Geometry: final body of the model. Coordinates: model frame, mm. A direction names the side the tool comes from. Give positions to 0.01 mm unless a question says otherwise; leave off trailing zeros. Write each loop counter-clockwise with the first axis right and the second up, starting at its lowest first coordinate (ties: lowest second). Pieces come first, ordered by that corner, then holes.
Q1. Line query: line 1 (Y direction, x = 11, z = -35); line 2 (Y direction, x = 27.5, z = 35); line 3 (Z direction, x = 8.5, y = 14.5). Output: solid intervals per line, ascending.
Q2. Section C-C (y = 21.5). State how many separate pieces and enclosed holes the cut face has, plus the area to 3 significant figures.
Q3. Mould query, pull axis Y, two halves, no side actions, for faces 1 (the flat face through (9, 27, 1)), 2 (the cylindrical face through (26.1, 5.2, 39.4)), 3 (the flat face through (22, 17, 35)), 4 (the flat face through (0, 13, 35)). Classes: +Y half, -Y half, draft (parallel to the pull), parting line (faces both ways), or undercut.
Q4. Section A-A (x = 25.5). Return the cut outline in (y, z), plus the area to 3 significant figures.
Q5. Pin query (flat end, axial travel): pin 1 Ø3 at (y, z) = (19, -5) entering from -X; pin 2 Ø10 at (y, z) = (20.5, -35) entering from +X; pin 3 Ø7.5 at (y, z) = (16.5, 3) entering from +X. Return the tip coordinate at first contact, or that it passes through.
Q6. Section D-D (z = 5). Return the cut outline in (x, y), plus the area to 3 significant figures.
Q7. Reachability of faces 5 (the flat face through (15, 20, 10.5)), 6 (the flat face through (4, 13, 25.25)), 7 (the flat face through (22, 21, -39)) from +Z, -Z, +X, -X, +Y, -Y: full face, straight path, thin tool, end or side. Return the list, or none.
Q8. Section B-B (z = 35). Return the cut outline in (x, y), plus the area to 3 significant figures.
Autodesk Inventor part; units mm, degrees
ref_plane "YZ Plane" through (0, 0, 0) normal (1, 0, 0) x (0, 1, 0)
ref_plane "XZ Plane" through (0, 0, 0) normal (0, 1, 0) x (-1, 0, 0)
ref_plane "XY Plane" through (0, 0, 0) normal (0, 0, 1) x (1, 0, 0)
sketch "Szkic2" plane through (0, 0, 0) normal (0, 1, 0) x (-1, 0, 0)
  line L0 (-5, 13) -> (-5, -13)
  line L1 (1, -20.25) -> (1, 20.25)
  line L2 (-8.0627, 14.7682) -> (-5, 13)
  line L3 (-5, 16.0869) -> (-5, 13) construction
  arc A0 (-8.0627, 14.7682) -> (-5, 16.0869) centre (-8.5, 20) ccw construction
  line L4 (-3.256, 20.25) -> (-5, 20.25) construction
  arc A1 (-5, 16.0869) -> (-3.256, 20.25) centre (-8.5, 20) ccw construction
  line L5 (1, 20.25) -> (-3.256, 20.25)
  line L6 (-5, 20.25) -> (-5, 16.0869) construction
  line L7 (-5, -13) -> (-8.0627, -14.7682)
  line L8 (-5, -13) -> (-5, -16.0869) construction
  arc A2 (-5, -16.0869) -> (-8.0627, -14.7682) centre (-8.5, -20) ccw construction
  line L9 (-3.256, -20.25) -> (1, -20.25)
  arc A3 (-3.256, -20.25) -> (-5, -16.0869) centre (-8.5, -20) ccw construction
  line L10 (-5, -16.0869) -> (-5, -20.25) construction
  line L11 (-5, -20.25) -> (-3.256, -20.25) construction
  arc A4 (-8.0627, -14.7682) -> (-3.256, -20.25) centre (-8.5, -20) ccw
  arc A5 (-3.256, 20.25) -> (-8.0627, 14.7682) centre (-8.5, 20) ccw
  line L12 (0, 45) -> (-30, 45)
  line L13 (-30, 45) -> (-30, -45)
  line L14 (-30, -45) -> (0, -45)
  line L15 (0, -45) -> (0, 45)
  line L16 (-8.5, 25.25) -> (0, 25.25)
  line L17 (-8.5, -25.25) -> (0, -25.25)
  point P0 (0, 0)
  point P1 (0, -20.25)
  point P2 (0, 20.25)
  dimension "d0" = 10.5
  dimension "d1" = 6
  dimension "d2" = 3.5
  dimension "d3" = 120
  dimension "d4" = 120
  dimension "d5" = 26
  dimension "d6" = 40
  dimension "d8" = 7
  dimension "d9" = 0.25
  dimension "d10" = 0.25
  dimension "d12" = 9.5
  dimension "d14" = 1
  dimension "d15" = 20
  dimension "d16" = 90
  dimension "d17" = 45
  dimension "d18" = 30
extrude "Wyciągnięcie proste1" add sketch "Szkic2" along normal blind 27 contours L0 L7 A4 L17 L15 L14 L13 L12 L16 A5 L2
sketch "Szkic3" plane through (30, 0, 45) normal (1, 0, 0) x (0, 0, -1)
  circle A0 centre (10, 20.5) radius 3.25
  circle A1 centre (10, 8.5) radius 3.25
  circle A2 centre (80, 20.5) radius 3.25
  circle A3 centre (80, 8.5) radius 3.25
  line L0 (0, 0) -> (0, 27)
  line L1 (0, 27) -> (90, 27)
  line L2 (90, 0) -> (90, 27)
  circle A4 centre (10, 20.5) radius 5.5
  circle A5 centre (10, 8.5) radius 5.5
  circle A6 centre (80, 20.5) radius 5.5
  circle A7 centre (80, 8.5) radius 5.5
  point P0 (45, 0)
  dimension "d21" = 6.5
  dimension "d22" = 10
  dimension "d23" = 6.5
  dimension "d24" = 12
  dimension "d25" = 10
  dimension "d26" = 11
extrude "Wyciągnięcie proste2" cut sketch "Szkic3" against normal through all contours A0 | A1 | A2 | A3
extrude "Wyciągnięcie proste3" cut sketch "Szkic3" against normal blind 8 contours A1 | A2 | A3 | A4 | A5 | A6 | A7
sketch "Szkic4" plane through (0, 27, 0) normal (0, 1, 0) x (1, 0, 0)
  line L0 (30, -45) -> (30, 45)
  circle A0 centre (38.5, 0) radius 22
  point P0 (0, 0)
  dimension "d34" = 44
  dimension "d37" = 8.5
  dimension "d38" = 38.5
extrude "Wyciągnięcie proste4" cut sketch "Szkic4" against normal through all
sketch "Szkic8" plane through (0, 27, 0) normal (0, 1, 0) x (1, 0, 0)
  line L0 (11, -10.5) -> (21, -10.5)
  line L1 (21, -10.5) -> (21, 10.5)
  line L2 (21, 10.5) -> (11, 10.5)
  line L3 (11, 10.5) -> (11, -10.5)
  line L4 (5, 13) -> (5, -13)
  point P0 (0, 0)
  dimension "d58" = 21
  dimension "d59" = 6
  dimension "d60" = 10.5
  dimension "d61" = 10
extrude "Wyciągnięcie proste8" cut sketch "Szkic8" against normal blind 15
sketch "Szkic9" plane through (11, 27, 10.5) normal (1, 0, 0) x (0, 0, -1)
  circle A0 centre (5.5, -8) radius 1
  circle A1 centre (15.5, -8) radius 1
  line L0 (0, 0) -> (21, 0)
  line L1 (0, -15) -> (0, 0)
  point P0 (10.5, -27)
  dimension "d64" = 2
  dimension "d65" = 10
  dimension "d66" = 8
  dimension "d67" = 5.5
extrude "Wyciągnięcie proste9" cut sketch "Szkic9" against normal through all
equation "\"d25\" = d22"
properties part number "YCarriageFrontHolder" material "Tworzywo sztuczne ABS"
Computed:
1. line 1: y = 0 to 5.25, 11.75 to 17.25, 23.75 to 27
1. line 2: y = 0 to 3, 14 to 15, 26 to 27
1. line 3: z = -45 to -25.25, -14.75 to 14.75, 25.25 to 45
2. separate pieces: 3
2. enclosed holes: 0
2. area: 1,310 mm2
3. face 1: +Y half
3. face 2: undercut
3. face 3: undercut
3. face 4: draft
4. outline: (0, -45) - (27, -45) - (27, -17.75) - (0, -17.75) - close; (0, 17.75) - (27, 17.75) - (27, 45) - (0, 45) - close; hole circle Ø11 at (8.5, -35); hole circle Ø11 at (8.5, 35); hole circle Ø11 at (20.5, -35); hole circle Ø11 at (20.5, 35)
4. area: 1,090 mm2
5. pin 1: stops at x = 5
5. pin 2: stops at x = 22
5. pin 3: stops at x = 11
6. outline: (5, 0) - (17.08, 0) - (17.08, 12) - (11, 12) - (11, 18) - (5, 18) - close; (5, 20) - (11, 20) - (11, 27) - (5, 27) - close
6. area: 223 mm2
7. face 5: +X, +Y
7. face 6: -X, +Y, -Y
7. face 7: +X
8. outline: (0, 0) - (30, 0) - (30, 3) - (22, 3) - (22, 5.25) - (0, 5.25) - close; (0, 11.75) - (22, 11.75) - (22, 14) - (30, 14) - (30, 15) - (22, 15) - (22, 17.25) - (0, 17.25) - close; (0, 23.75) - (22, 23.75) - (22, 26) - (30, 26) - (30, 27) - (0, 27) - close
8. area: 348 mm2
